```python
from build123d import *

# Parameters (mm, degrees)
BOSS_EXTRUDE1_DEPTH = 12.7
SKETCH2_R           = 5.5
SKETCH2_R_2         = 4.1
BOSS_EXTRUDE2_DEPTH = 3.499999906
CIRPATTERN1_COUNT   = 3
SKETCH6_R           = 4
CUT_EXTRUDE1_DEPTH  = 17.199999906
RANDOM_CIRCLES_R    = 2.3
CUT_EXTRUDE2_DEPTH  = 2.54
SKETCH8_R           = 2.5
BOSS_EXTRUDE3_DEPTH = 25.4


with BuildPart() as part:
    # Sketch1 → Boss-Extrude1 (new body)
    with BuildSketch(Plane(origin=(0, 0, 0), x_dir=(1, 0, 0), z_dir=(0, 1, 0))):
        Polygon((11.547005384, -20), (23.094010768, 0), (11.547005384, 20), (-11.547005384, 20), (-23.094010768, 0), (-11.547005384, -20), align=None)
    extrude(amount=BOSS_EXTRUDE1_DEPTH)

    # Sketch2 → Boss-Extrude2 (add)
    with BuildSketch(Plane.XZ):
        Circle(SKETCH2_R)
        Circle(SKETCH2_R_2, mode=Mode.SUBTRACT)
    extrude(amount=BOSS_EXTRUDE2_DEPTH)

    # Sketch5 → Cut-Revolve1 (revolve, cut)
    with BuildSketch(Plane(origin=(0, 12.7, 0), x_dir=(1, 0, 0), z_dir=(0, 1, 0))):
        Polygon((0, -20), (0, -4.792), (-3.81, -4.792), (-3.81, -10.888), (-11.176, -10.888), (-11.176, -18), (-6.5, -18), (-6.5, -20), align=None)
    cut_revolve1 = revolve(axis=Axis((0, 12.7, 20), (0, 0, -1)), mode=Mode.SUBTRACT)

    # CirPattern1: Cut-Revolve1 ×3 about axis
    cirpattern1_axis = Axis((0, 0, 0), (0, 1, 0))
    for i in range(1, CIRPATTERN1_COUNT):
        add(cut_revolve1.rotate(cirpattern1_axis, i * 360 / CIRPATTERN1_COUNT), mode=Mode.SUBTRACT)

    # Sketch6 → Cut-Extrude1 (cut, through all)
    with BuildSketch(Plane(origin=(0, 12.7, 0), x_dir=(1, 0, 0), z_dir=(0, 1, 0))):
        Circle(SKETCH6_R)
    extrude(amount=-CUT_EXTRUDE1_DEPTH, mode=Mode.SUBTRACT)

    # Random Circles → Cut-Extrude2 (cut)
    with BuildSketch(Plane(origin=(0, 12.7, 0), x_dir=(1, 0, 0), z_dir=(0, 1, 0))):
        with Locations((0, 14.7)):
            Circle(RANDOM_CIRCLES_R)
        with Locations((12.730569972, -7.350006)):
            Circle(RANDOM_CIRCLES_R)
        with Locations((-12.730580364, -7.35)):
            Circle(RANDOM_CIRCLES_R)
    extrude(amount=-CUT_EXTRUDE2_DEPTH, mode=Mode.SUBTRACT)

    # Sketch8 → Boss-Extrude3 (add)
    with BuildSketch(Plane(origin=(0, 0, 0), x_dir=(1, 0, 0), z_dir=(0, 1, 0))):
        with Locations((0, 16.40962)):
            Circle(SKETCH8_R)
        with Locations((14.211147786, -8.20481)):
            Circle(SKETCH8_R)
        with Locations((-14.211147786, -8.20481)):
            Circle(SKETCH8_R)
    extrude(amount=-BOSS_EXTRUDE3_DEPTH)


solid = part.part
```
For this review, take the finished solid that the model builds, in its own axes (mm). A direction names the side the tool comes from. Round coordinates to 2 decimals unless told otherwise and drop trailing zeros. Loops run counter-clockwise (first coordinate to the right, second up) from the corner with the lowest first, then second, coordinate; pieces in that order, holes last.
Q1. To check wall thickness, follow line 1 along Z through (x, y) = (0, 5); line 2 along Z through (x, y) = (0, -1.2); line 3 along Z through (x, y) = (0, 7). State the ranges of each line that lie inside material, in increasing order.
Result sheet:
line 1: z = -20 to -4, 4 to 10.89, 18 to 20
line 2: z = -18.91 to -13.91, -5.5 to -4.1, 4.1 to 5.5
line 3: z = -20 to -4, 4 to 10.89
Q2. Mouldability with a two-part tool opening along X and no side actions: class faces 4 (the face through (17.4, 4.85, -9.86)), 5 (the face through (-6.87, 8.89, -3.87)), 6 (the face through (-17.4, 6.26, 9.86)) as +X half, -X half, draft (parallel to the pull), parting line (faces both ways), or undercut.
Result sheet:
face 4: +X half
face 5: undercut
face 6: -X half
Q3. Add section D-D on y = -15. Write out the cut boundary in (x, z).
Result sheet:
outline: circle Ø5 at (-14.21, 8.2); circle Ø5 at (0, -16.41); circle Ø5 at (14.21, 8.2)
Q4. Insertion check: pin 1 Ø20 at (x, z) = (4.5, -8.5) entering from -Y; pin 2 Ø10 at (x, y) = (-14, -17) entering from -Z; pin 3 Ø3 at (x, z) = (0, -14.7) entering from +Y; pin 4 Ø4 at (x, z) = (-13.5, -10) entering from -Y. Each pin has a flat end and moves straight along its axis. Give the tip position at first contact, or say it passes through.
Result sheet:
pin 1: stops at y = -25.4
pin 2: stops at z = 5.7
pin 3: stops at y = 10.16
pin 4: stops at y = 0
Q5. Machinability: for faces 1 (the face through (0, 6, -20)), 2 (the face through (-16.195, -12.522, 9.726)), 3 (the face through (0, 11, -17)), which of the approach directions +Z, -Z, +X, -X, +Y, -Y give a long, thin tool a straight path to every point of the face, cutting with its end or side? Answer none if there is none.
Result sheet:
face 1: -Z, +X, -X, +Y, -Y
face 2: -Y
face 3: +Y
Q6. Add section B-B on y = -2. Write out the cut boundary in (x, z).
Result sheet:
outline: circle Ø5 at (-14.21, 8.2); circle Ø11 at (0, 0); circle Ø5 at (0, -16.41); circle Ø5 at (14.21, 8.2); hole circle Ø8.2 at (0, 0)
